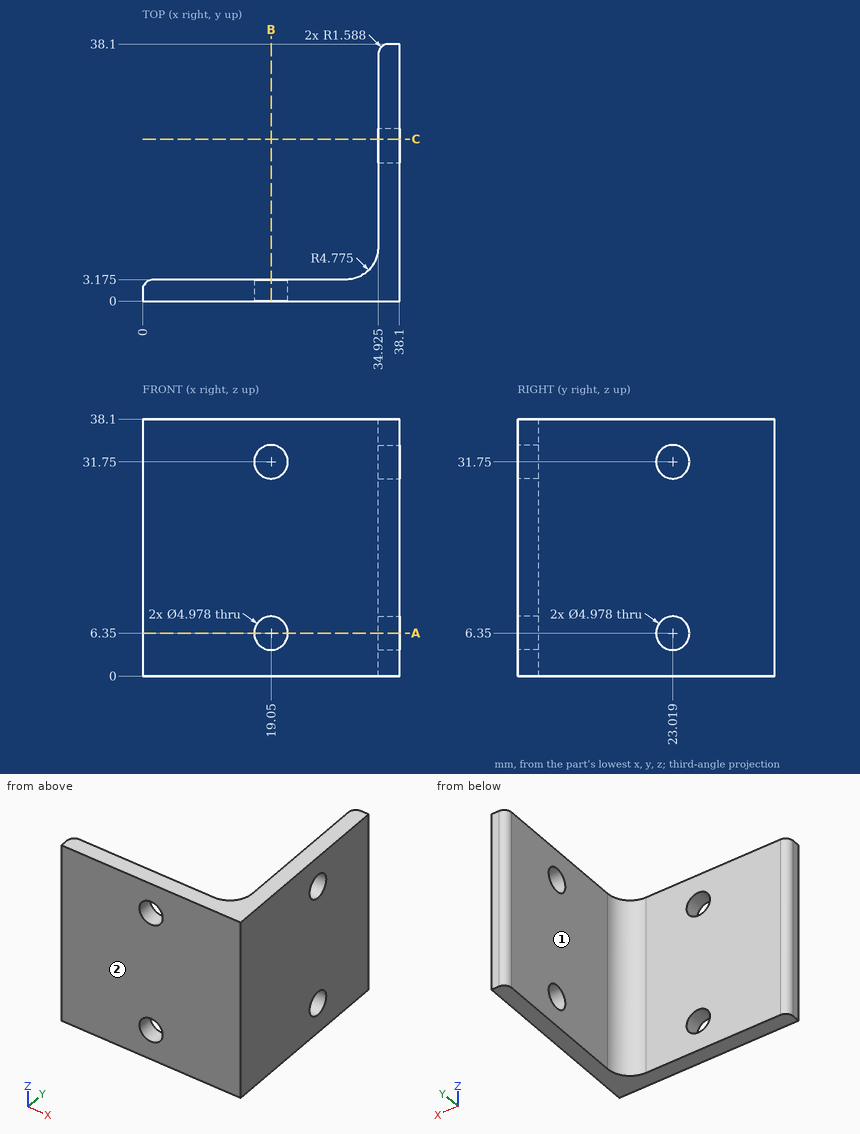
For this review, use the dimensioned drawing (mm, ordinates from the lowest corner) and the shaded views. A direction names the side the tool comes from. Round coordinates to 2 decimals unless told otherwise and drop trailing zeros. Write each loop counter-clockwise with the first axis right and the second up, starting at its lowest first coordinate (ties: lowest second). Pieces come first, ordered by that corner, then holes. Notation, with made-up numbers: (46.5, 12) - (55.5, 12) arc R13 cw to (55.5, 18) - close; hole circle Ø8 at (-7.5, -23.75). An arc over 180 degrees is marked (long way). Answer as a JSON object with one key per item and string values.
1. Tool access review of the marked faces 1 and 2: name each direction out of +Z, -Z, +X, -X, +Y, -Y from which nothing blocks a thin tool from reaching the whole face with its end or side.
Response values:
{"face 1": "+Z, -Z, -X, +Y", "face 2": "+Z, -Z, +X, -X, -Y"}
2. To check wall thickness, follow line 1 along Z through (x, y) = (19.05, 0.7); line 2 along Y through (x, z) = (14, 33.5) (1 decimal); line 3 along Y through (x, z) = (36, 31) (1 decimal). State the ranges of each line that lie inside material, in increasing order.
Response values:
{"line 1": "z = 0 to 3.86, 8.84 to 29.26, 34.24 to 38.1", "line 2": "y = 0 to 3.2", "line 3": "y = 0 to 20.6, 25.4 to 38"}
3. We need section A-A on z = 6.35. Count the separate pieces of the cut face and the enclosed holes in it, then the cut area to 3 significant figures.
Response values:
{"separate pieces": "3", "enclosed holes": "0", "area": "204 mm2"}
4. We need section C-C on y = 24. Give the boundary of the cut face in (x, z) (1 decimal).
Response values:
{"outline": "(34.9, 0) - (38.1, 0) - (38.1, 4.1) - (34.9, 4.1) - close; (34.9, 8.6) - (38.1, 8.6) - (38.1, 29.5) - (34.9, 29.5) - close; (34.9, 34) - (38.1, 34) - (38.1, 38.1) - (34.9, 38.1) - close"}
5. We need section B-B on x = 19.05. Give the boundary of the cut face in (y, z) (1 decimal).
Response values:
{"outline": "(0, 0) - (3.2, 0) - (3.2, 3.9) - (0, 3.9) - close; (0, 8.8) - (3.2, 8.8) - (3.2, 29.3) - (0, 29.3) - close; (0, 34.2) - (3.2, 34.2) - (3.2, 38.1) - (0, 38.1) - close"}
6. For pin 1 Ø14.5 at (x, z) = (21.5, 12.5) entering from +Y (1 decimal); pin 2 Ø3 at (x, y) = (32, 29.5) entering from -Z; pin 3 Ø2 at (y, z) = (13.5, 8.5) entering from -X (1 decimal), all flat-tipped, find the tip position at first contact; note any pin that passes through.
Response values:
{"pin 1": "stops at y = 3.2", "pin 2": "passes through", "pin 3": "stops at x = 34.9"}
